from build123d import *

# Parameters (mm, degrees)
F1_DEPTH  = 8
F2_DEPTH  = 5.92
F3_R      = 3
F4_R      = 5
F6_DEPTH  = 20.601
F8_DEPTH  = 20.6010001
F9_R      = 1
F11_DEPTH = 1


with BuildPart() as f1:
    # F0 (on Top) → F1 (new body)
    with BuildSketch(Plane.XY):
        with BuildLine():
            Line((-20, 20.6), (-20, 0))
            Line((-20, 0), (-8.03, 0))
            ThreePointArc((-8.03, 0), (0, 8.03), (8.03, 0))
            Line((8.03, 0), (20, 0))
            Line((20, 0), (20, 20.6))
            Line((20, 20.6), (-20, 20.6))
        make_face()
    extrude(amount=-F1_DEPTH)

    # F0 (on Top) → F2 (join)
    with BuildSketch(Plane.XY):
        with BuildLine():
            ThreePointArc((8.03, 0), (0, 8.03), (-8.03, 0))
            Line((-8.03, 0), (-6.02, 0))
            ThreePointArc((-6.02, 0), (0, 6.02), (6.02, 0))
            Line((6.02, 0), (8.03, 0))
        make_face()
    extrude(amount=-F2_DEPTH)

    # F3
    f3_edges = [f1.edges().sort_by_distance(p)[0] for p in [
        (0, 20.6, 0),
    ]]
    fillet(f3_edges, radius=F3_R)

    # F4
    f4_edges = [f1.edges().sort_by_distance(p)[0] for p in [
        (-20, 0, -4),
        (20, 0, -4),
    ]]
    fillet(f4_edges, radius=F4_R)

    # F5 (on face) → F6 (cut, through all)
    with BuildSketch(Plane.XZ):
        with BuildLine():
            Line((-15, -5.6), (-15, -2.4))
            ThreePointArc((-15, -2.4), (-16.6, -4), (-15, -5.6))
        make_face()
        with BuildLine():
            ThreePointArc((-15, -5.6), (-13.8686291501, -5.1313708499), (-13.4, -4))
            ThreePointArc((-13.4, -4), (-13.8686291501, -2.8686291501), (-15, -2.4))
            Line((-15, -2.4), (-15, -5.6))
        make_face()
    extrude(amount=-F6_DEPTH, mode=Mode.SUBTRACT)

    # F7 (on face) → F8 (cut, through all)
    with BuildSketch(Plane.XZ):
        with BuildLine():
            Line((15, -5.6), (15, -2.4))
            ThreePointArc((15, -2.4), (13.4, -4), (15, -5.6))
        make_face()
        with BuildLine():
            ThreePointArc((15, -5.6), (16.1313708499, -5.1313708499), (16.6, -4))
            ThreePointArc((16.6, -4), (16.1313708499, -2.8686291501), (15, -2.4))
            Line((15, -2.4), (15, -5.6))
        make_face()
    extrude(amount=-F8_DEPTH, mode=Mode.SUBTRACT)

    # F9
    f9_edges = [f1.edges().sort_by_distance(p)[0] for p in [
        (-8.03, 0, -6.96),
        (-6.02, 0, -2.96),
        (6.02, 0, -2.96),
        (8.03, 0, -6.96),
    ]]
    fillet(f9_edges, radius=F9_R)

    # F10 (on face) → F11 (cut)
    with BuildSketch(Plane(origin=(0, 20.6, 0), x_dir=(-1, 0, 0), z_dir=(0, 1, 0))):
        with BuildLine():
            Line((-13.7510004003, -3), (-12.0657198498, -3))
            ThreePointArc((-12.0657198498, -3), (-15, -0.9), (-17.9342801502, -3))
            Line((-17.9342801502, -3), (-16.2489995997, -3))
            ThreePointArc((-16.2489995997, -3), (-16.4422205102, -4.692820323), (-15, -5.6))
            ThreePointArc((-15, -5.6), (-13.5577794898, -4.692820323), (-13.7510004003, -3))
        make_face()
        with BuildLine():
            ThreePointArc((-17.9342801502, -3), (-15.5068192648, -7.0582894292), (-11.9, -4))
            ThreePointArc((-11.9, -4), (-11.9417105708, -3.4931807352), (-12.0657198498, -3))
            Line((-12.0657198498, -3), (-13.7510004003, -3))
            ThreePointArc((-13.7510004003, -3), (-13.5577794898, -4.692820323), (-15, -5.6))
            ThreePointArc((-15, -5.6), (-16.4422205102, -4.692820323), (-16.2489995997, -3))
            Line((-16.2489995997, -3), (-17.9342801502, -3))
        make_face()
        with BuildLine():
            ThreePointArc((17.9342801502, -3), (15, -0.9), (12.0657198498, -3))
            Line((12.0657198498, -3), (13.7510004003, -3))
            ThreePointArc((13.7510004003, -3), (13.5577794898, -4.692820323), (15, -5.6))
            ThreePointArc((15, -5.6), (16.4422205102, -4.692820323), (16.2489995997, -3))
            Line((16.2489995997, -3), (17.9342801502, -3))
        make_face()
        with BuildLine():
            Line((13.7510004003, -3), (12.0657198498, -3))
            ThreePointArc((12.0657198498, -3), (14.4931807352, -7.0582894292), (18.1, -4))
            ThreePointArc((18.1, -4), (18.0582894292, -3.4931807352), (17.9342801502, -3))
            Line((17.9342801502, -3), (16.2489995997, -3))
            ThreePointArc((16.2489995997, -3), (16.4422205102, -4.692820323), (15, -5.6))
            ThreePointArc((15, -5.6), (13.5577794898, -4.692820323), (13.7510004003, -3))
        make_face()
    extrude(amount=-F11_DEPTH, mode=Mode.SUBTRACT)


solid = f1.part
Geometry check sheet. Reference: the model listing, model coordinates, mm. A direction names the side the tool comes from. Round coordinates to 2 decimals unless told otherwise and drop trailing zeros. Write each loop counter-clockwise with the first axis right and the second up, starting at its lowest first coordinate (ties: lowest second). Pieces come first, ordered by that corner, then holes. Notation, with made-up numbers: (-0.75, -23) -> (51.25, -23) arc R16 cw to (51.25, -7) -> close; hole circle Ø6 at (-8, 70). An arc over 180 degrees is marked (long way). One line per item, written item: value. Start each with the question number.
(1) Draft check along X on faces 5 (the flat face through (20, 13, -4)), 6 (the flat face through (0, 20.6, -6)), 7 (the cylindrical face through (6.3, 0.24, -3)). Enter one of: +X half, -X half, draft (parallel to the pull), parting line (faces both ways), or undercut.
(2) Go/stop test with flat-tipped pins: pin 1 Ø3 at (y, z) = (2.5, -5.5) entering from -X; pin 2 Ø3.5 at (x, z) = (15, -4) entering from +Y; pin 3 Ø2.5 at (x, y) = (-4.5, 3) entering from -Z. Record where each tip stops, or that it passes through.
(3) Scan lines: line 1 (X direction, y = 20.2, z = -4); line 2 (X direction, y = 16, z = -4); line 3 (Y direction, x = 0, z = -7.5). Record each from-to range of solid material in increasing order. Write a range as [from, to].
(4) Cross-section at C-C, the plane x = -14. Record the cut outline in (y, z), and give its area (3 significant figures).
(5) Access from +Z, -Z, +X, -X, +Y, -Y to the whole of each face (thin tool, end or side, straight path). Record for faces 1 (the flat face through (13.7, 19.6, -5.3)), 2 (the flat face through (-0.7, 6.4, -5.92)), 3 (the flat face through (-20, 13, -4)), 4 (the cylindrical face through (-6.3, 0.24, -3)).
(6) Cross-section at B-B, the plane y = 10.25. Record the cut outline in (x, z), and give its area (3 significant figures).
(7) Cross-section at A-A, the plane y = 1.75. Record the cut outline in (x, z), and give its area (3 significant figures).
(8) Cross-section at D-D, the plane z = -1.5. Record the cut outline in (x, y), and give its area (3 significant figures).
Answer:
1. face 5: +X half
1. face 6: draft
1. face 7: undercut
2. pin 1: x = -19.9
2. pin 2: y = 19.6
2. pin 3: z = -5.92
3. line 1: [-20, -18.1], [-11.9, 11.9], [18.1, 20]
3. line 2: [-20, -16.6], [-13.4, 13.4], [16.6, 20]
3. line 3: [8.03, 20.6]
4. outline: (0, -8) -> (20.6, -8) -> (20.6, -6.93) -> (19.6, -6.93) -> (19.6, -5.25) -> (0, -5.25) -> close; (0, -2.75) -> (19.6, -2.75) -> (19.6, -1.07) -> (19.89, -1.07) arc R3 ccw to (17.6, 0) -> (0, 0) -> close
4. area: 108 mm²
5. face 1: +Y
5. face 2: -Z, -Y
5. face 3: +Z, -Z, -X, +Y, -Y
5. face 4: +Z, -Z, -Y
6. outline: (-20, -8) -> (20, -8) -> (20, 0) -> (-20, 0) -> close; hole circle Ø3.2 at (-15, -4); hole circle Ø3.2 at (15, -4)
6. area: 304 mm²
7. outline: (-18.8, -8) -> (-7.84, -8) -> (-7.84, -5.92) -> (-5.76, -5.92) -> (-5.76, 0) -> (-18.8, 0) -> close; (5.76, -5.92) -> (7.84, -5.92) -> (7.84, -8) -> (18.8, -8) -> (18.8, 0) -> (5.76, 0) -> close; hole circle Ø3.2 at (-15, -4); hole circle Ø3.2 at (15, -4)
7. area: 184 mm²
8. outline: (-20, 5) arc R5 ccw to (-15, 0) -> (-6.95, 0) arc R1 ccw to (-5.96, 0.86) arc R6.02 cw to (5.96, 0.86) arc R1 ccw to (6.95, 0) -> (15, 0) arc R5 ccw to (20, 5) -> (20, 20.2) -> (16.83, 20.2) -> (16.83, 19.6) -> (13.17, 19.6) -> (13.17, 20.2) -> (-13.17, 20.2) -> (-13.17, 19.6) -> (-16.83, 19.6) -> (-16.83, 20.2) -> (-20, 20.2) -> close
8. area: 736 mm²
